Design review of the part built by this model. Coordinates are the model's own, in mm. A direction names the side the tool comes from. Round coordinates to 2 decimals unless told otherwise and drop trailing zeros. Loops run counter-clockwise (first coordinate to the right, second up) from the corner with the lowest first, then second, coordinate; pieces in that order, holes last. Notation, with made-up numbers: (21.25, -11.5) -> (37.25, -11.5) arc R34 cw to (37.25, 21.5) -> close; hole circle Ø11 at (17.5, 45). An arc over 180 degrees is marked (long way). Write each question's results on one line, items separated by ' | '. Start each with the question number.
from build123d import *
from build123d.topology import SkipClean

# Parameters (mm, degrees)
SKETCH_1_R       = 16.5
SKETCH_1_R_2     = 4
EXTRUDE_4_DEPTH  = 3
EXTRUDE_6_DEPTH  = 10
EXTRUDE_12_DEPTH = 3
EXTRUDE_14_DEPTH = 3.2


with BuildPart() as part:
    # 草图1 → 凸台-拉伸4 (new body)
    with BuildSketch(Plane.XY):
        with Locations((0, 3e-09)):
            Circle(SKETCH_1_R)
        with Locations((0, 3e-09)):
            Circle(SKETCH_1_R_2, mode=Mode.SUBTRACT)
        with BuildLine():
            Line((-7.017492281, 9.175302033), (-4.189065156, 6.346874908))
            ThreePointArc((-4.189065156, 6.346874908), (-4.189065156, 4.154843887), (-6.381096178, 4.154843887))
            Line((-6.381096178, 4.154843887), (-9.209523303, 6.983271012))
            ThreePointArc((-9.209523303, 6.983271012), (-9.209523303, 9.175302033), (-7.017492281, 9.175302033))
        make_face(mode=Mode.SUBTRACT)
        with BuildLine():
            Line((7.017492281, 9.209523305), (4.189065156, 6.381096181))
            ThreePointArc((4.189065156, 6.381096181), (4.189065156, 4.189065159), (6.381096178, 4.189065159))
            Line((6.381096178, 4.189065159), (9.209523303, 7.017492284))
            ThreePointArc((9.209523303, 7.017492284), (9.209523303, 9.209523305), (7.017492281, 9.209523305))
        make_face(mode=Mode.SUBTRACT)
        with BuildLine():
            Line((-7.017492281, -9.2095233), (-4.189065156, -6.381096175))
            ThreePointArc((-4.189065156, -6.381096175), (-4.189065156, -4.189065153), (-6.381096178, -4.189065153))
            Line((-6.381096178, -4.189065153), (-9.209523303, -7.017492278))
            ThreePointArc((-9.209523303, -7.017492278), (-9.209523303, -9.2095233), (-7.017492281, -9.2095233))
        make_face(mode=Mode.SUBTRACT)
        with BuildLine():
            Line((7.017492281, -9.2095233), (4.189065156, -6.381096175))
            ThreePointArc((4.189065156, -6.381096175), (4.189065156, -4.189065153), (6.381096178, -4.189065153))
            Line((6.381096178, -4.189065153), (9.209523303, -7.017492278))
            ThreePointArc((9.209523303, -7.017492278), (9.209523303, -9.2095233), (7.017492281, -9.2095233))
        make_face(mode=Mode.SUBTRACT)
    extrude(amount=EXTRUDE_4_DEPTH)

    # 草图3 → 凸台-拉伸6 (add)
    with SkipClean():  # the faces are left unmerged after this step: merging them gives an invalid solid
        with BuildSketch(Plane.XY.offset(3)):
            with BuildLine():
                Line((16.422241017, 1.600000001), (3.666060557, 1.600000001))
                ThreePointArc((3.666060557, 1.600000001), (4, 0), (3.666060555, -1.6))
                Line((3.666060555, -1.6), (16.422241016, -1.6))
                ThreePointArc((16.422241016, -1.6), (16.5, 0), (16.422241017, 1.600000001))
            make_face()
            with BuildLine():
                Line((-16.422241017, 1.600000001), (-3.666060557, 1.600000001))
                ThreePointArc((-3.666060557, 1.600000001), (-4, 0), (-3.666060555, -1.6))
                Line((-3.666060555, -1.6), (-16.422241016, -1.6))
                ThreePointArc((-16.422241016, -1.6), (-16.5, 0), (-16.422241017, 1.600000001))
            make_face()
        extrude(amount=EXTRUDE_6_DEPTH)

    # 草图4 → 凸台-拉伸12 (add)
    with SkipClean():  # the faces are left unmerged after this step: merging them gives an invalid solid
        with BuildSketch(Plane.XY.offset(13)):
            with BuildLine():
                Line((-16.422241017, 1.600000001), (16.422241017, 1.600000001))
                ThreePointArc((16.422241017, 1.600000001), (16.5, 0), (16.422241016, -1.6))
                Line((16.422241016, -1.6), (-16.422241016, -1.6))
                ThreePointArc((-16.422241016, -1.6), (-16.5, 0), (-16.422241017, 1.600000001))
            make_face()
        extrude(amount=EXTRUDE_12_DEPTH)

    # 草图8 → 凸台-拉伸14 (add)
    with SkipClean():  # the faces are left unmerged after this step: merging them gives an invalid solid
        with BuildSketch(Plane(origin=(0, 1.600000001, 0), x_dir=(1, 0, 0), z_dir=(0, 1, 0))):
            with BuildLine():
                Line((-16.422241017, -16), (-16.422241017, -55.152668259))
                ThreePointArc((-16.422241017, -55.152668259), (-14.570166648, -58.527044569), (-10.729033275, -58.776622942))
                ThreePointArc((-10.729033275, -58.776622942), (9.115230867, -41.353795196), (16.5, -16))
                Line((16.5, -16), (-16.422241017, -16))
            make_face()
            with BuildLine():
                Line((-6.919334161, -22.910583914), (4.502935407, -22.910583914))
                ThreePointArc((4.502935407, -22.910583914), (7.555031335, -24.325103215), (8.448502964, -27.568228691))
                ThreePointArc((8.448502964, -27.568228691), (3.06689673, -40.042318745), (-7.503409516, -48.576557679))
                ThreePointArc((-7.503409516, -48.576557679), (-9.80808954, -48.426810655), (-10.919334161, -46.402184869))
                Line((-10.919334161, -46.402184869), (-10.919334161, -26.910583914))
                ThreePointArc((-10.919334161, -26.910583914), (-9.747761286, -24.082156789), (-6.919334161, -22.910583914))
            make_face(mode=Mode.SUBTRACT)
        extrude(amount=-EXTRUDE_14_DEPTH)


solid = part.part
1) Take a section at C-C (x = 0.5). Write out the cut boundary in (y, z).
2) To check wall thickness, follow line 1 (Y direction, x = 0, z = 2); line 2 (Z direction, x = 13, y = 8.5); line 3 (Z direction, x = 6.5, y = 1). State the ranges of each line that lie inside material, in increasing order. Write a range as from..to.
3) For faces 1 (the face through (-7.776, 5.549, 1.479)), 2 (the face through (-9.779, 0.022, 24.113)), 3 (the face through (0, -7, 3)), 4 (the face through (3, -3, 0)), 5 (the face through (-4, 1.6, 18)), list the 3-axis set-ups (+Z, -Z, +X, -X, +Y, -Y) from which the entire face can be reached by the end or side of a thin tool; tool diameter is ignored.
4) Take a section at A-A (z = 7). Write out the cut boundary in (x, y).
5) Take a section at D-D (z = 15). Write out the cut boundary in (x, y), plus the area to 3 significant figures.
6) The part is to be moulded in two halves that separate along Z. For faces 6 (the face through (7.776, -5.583, 1.479)), 7 (the face through (-10.919, 0, 37)), 8 (the face through (0, 0, 13)), 9 (the face through (-14.617, 0.022, 58.497)), say which applies: +Z half, -Z half, draft (parallel to the pull), parting line (faces both ways), or undercut.
7) Take a section at B-B (y = 2.5). Write out the cut boundary in (x, z).
8) Insertion check: pin 1 (13 mm diameter, centred on x = 0, y = 0, fed in from -Z); pin 2 (2 mm diameter, centred on x = -8.5, y = -3.5, fed in from +Z); pin 3 (5 mm diameter, centred on x = -13, z = 28, fed in from -Y); pin 4 (16.5 mm diameter, centred on x = 4, z = 32.5, fed in from +Y). Each pin has a flat end and moves straight along its axis. Give the tip position at first contact, or say it passes through.
Geometry check:
1) outline: (-16.49, 0) -> (-3.97, 0) -> (-3.97, 3) -> (-16.49, 3) -> close; (-1.6, 13) -> (1.6, 13) -> (1.6, 22.91) -> (-1.6, 22.91) -> close; (-1.6, 42.98) -> (1.6, 42.98) -> (1.6, 51.42) -> (-1.6, 51.42) -> close; (3.97, 0) -> (16.49, 0) -> (16.49, 3) -> (3.97, 3) -> close
2) line 1: y = -16.5..-4, 4..16.5 | line 2: z = 0..3 | line 3: z = 0..23.44, 34.17..45.06
3) face 1: +Z, -Z | face 2: +Y, -Y | face 3: +Z, +X, -X, -Y | face 4: -Z, +X, -X, +Y, -Y | face 5: +Z, +X, -X, +Y
4) outline: (-16.42, -1.6) -> (-3.67, -1.6) arc R4 cw to (-3.67, 1.6) -> (-16.42, 1.6) arc R16.5 ccw to start; (3.67, -1.6) -> (16.42, -1.6) arc R16.5 ccw to (16.42, 1.6) -> (3.67, 1.6) arc R4 cw to start
5) outline: (-16.42, -1.6) -> (16.42, -1.6) arc R16.5 ccw to (16.42, 1.6) -> (-16.42, 1.6) arc R16.5 ccw to start | area: 105 mm^2
6) face 6: draft | face 7: undercut | face 8: -Z half | face 9: +Z half
7) outline: (-16.31, 0) -> (-3.12, 0) -> (-3.12, 3) -> (-16.31, 3) -> close; (3.12, 0) -> (16.31, 0) -> (16.31, 3) -> (3.12, 3) -> close
8) pin 1: stops at z = 0 | pin 2: stops at z = 3 | pin 3: stops at y = -1.6 | pin 4: stops at y = 1.6
